Work out the finished part from the listing and answer in its coordinate system (mm). A direction names the side the tool comes from. Give positions to 0.01 mm unless a question says otherwise; leave off trailing zeros. Write each loop counter-clockwise with the first axis right and the second up, starting at its lowest first coordinate (ties: lowest second). Pieces come first, ordered by that corner, then holes. Notation, with made-up numbers: (-20, 46) -> (2, 46) arc R21 cw to (2, 75) -> close; hole circle Ø4 at (56, 3). An arc over 180 degrees is marked (long way). Use a Markdown table: item, result. Add a question column.
Q1. Section A-A, the plane y = 94.5 is taken. Give the vertices of the cut face in (x, z).
Q2. For faces 5 (the face through (0, 50, 0)), 6 (the face through (0, 55, 0)), 7 (the face through (-5.536, 10.14, 0.325)), 8 (the face through (0, 175, 8)), determine the directions among +Z, -Z, +X, -X, +Y, -Y from which every point of the face is accessible in a straight line to the end or side of a thin tool.
Q3. Consider line 1 (Z direction, x = 0, y = 69.75); line 2 (Z direction, x = 0, y = 4.5); line 3 (X direction, y = 84.5, z = 0.5). Determine where each line is inside the solid, lowest interval first.
Q4. For a pull along X with two mould halves and no side action, classify faces 1 (the face through (-2, 55, 6)), 2 (the face through (-1.08, 34.79, -4.88)), 3 (the face through (0, 0, 0)), 4 (the face through (1, 75, -5)) as pulls with the +X half, pulls with the -X half, needs draft (parallel to the pull), parting line crosses it, or undercut.
Q5. Each of these flat-tipped pins is pushed along its axis until it touches: pin 1 Ø1.8 at (x, z) = (0.5, 0.5) entering from +Y; pin 2 Ø10 at (y, z) = (132.5, -8.5) entering from -X; pin 3 Ø1.5 at (x, y) = (-1.5, 44) entering from -Z. Where does it stop, or does it pass through?
Autodesk Inventor part; units mm, degrees
ref_plane "YZ Plane" through (0, 0, 0) normal (1, 0, 0) x (0, 1, 0)
ref_plane "XZ Plane" through (0, 0, 0) normal (0, 1, 0) x (-1, 0, 0)
ref_plane "XY Plane" through (0, 0, 0) normal (0, 0, 1) x (1, 0, 0)
sketch "Sketch1" plane through (0, 0, 0) normal (0, 1, 0) x (-1, 0, 0)
  ellipse E0 centre (0, 0) end of major axis (0, 11.8) minor radius 4.3
  ellipse E1 centre (0, 0) end of major axis (11.8, 0) minor radius 4.3
  dimension "d0" = 11.8
  dimension "d1" = 4.3
  dimension "d2" = 11.8
  dimension "d3" = 4.3
sketch "Sketch2" plane through (0, 0, 0) normal (0, 1, 0) x (-1, 0, 0)
  circle A0 centre (7, 0) radius 1.5
  circle A1 centre (0, -7) radius 1.5
  circle A2 centre (-7, 0) radius 1.5
  circle A3 centre (0, 7) radius 1.5
  point P0 (0, 0)
  dimension "d4" = 3
  dimension "d5" = 3
  dimension "d6" = 3
  dimension "d7" = 3
  dimension "d8" = 7
  dimension "d9" = 7
  dimension "d10" = 7
  dimension "d11" = 7
extrude "Extrusion1" add sketch "Sketch1" along normal blind 20
hole "Hole1" at (7, 0, 0) at (0, 0, 7) at (0, 0, -7) at (-7, 0, 0) direction (0, 1, 0) diameter 3 depth 20 tip angle 118
sketch "Sketch5" plane through (0, 20, 0) normal (0, 1, 0) x (1, 0, 0)
  circle A0 centre (0, 0) radius 5
  circle A1 centre (0, 0) radius 3
  dimension "d25" = 10
  dimension "d26" = 6
extrude "Extrusion3" add sketch "Sketch5" along normal blind 30
sketch "Sketch6" plane through (0, 50, 0) normal (0, 1, 0) x (1, 0, 0)
  point P0 (0, 0)
sketch "Sketch7" plane through (0, 50, 0) normal (0, 1, 0) x (1, 0, 0)
  circle A0 centre (0, 0) radius 8
  dimension "d29" = 16
extrude "Extrusion4" add sketch "Sketch7" along normal blind 5
fillet "Fillet1" radius 6.7625 1 edges at (-8, 50, 0)
sketch "Sketch8" plane through (0, 55, 0) normal (0, 1, 0) x (1, 0, 0)
  circle A0 centre (0, 0) radius 8.5
  circle A1 centre (0, 0) radius 7.5
  dimension "d33" = 17
  dimension "d34" = 15
sketch "Sketch9" plane through (0, 55, 0) normal (0, 1, 0) x (1, 0, 0)
  circle A0 centre (0, 0) radius 5.75
  circle A1 centre (0, 0) radius 4.75
  dimension "d35" = 11.5
  dimension "d36" = 9.5
extrude "Extrusion5" add sketch "Sketch8" along normal blind 120
extrude "Extrusion6" add sketch "Sketch9" along normal blind 20
sketch "Sketch10" plane through (0, 75, 0) normal (0, 1, 0) x (1, 0, 0)
  point P0 (0, 0)
sketch "Sketch11" plane through (0, 75, 0) normal (0, 1, 0) x (1, 0, 0)
  point P0 (0, 0)
fillet "Fillet4" radius 2 1 edges at (-8.5, 55, 0)
properties part number "BB-8_headslider_stilt"
Result set:
| question | item | result |
|---|---|---|
| 1 | outline | circle Ø17 at (0, 0); hole circle Ø15 at (0, 0) |
| 2 | face 5 | none |
| 2 | face 6 | +Y |
| 2 | face 7 | -Y |
| 2 | face 8 | +Z, -Z, +X, -X, +Y |
| 3 | line 1 | z = -8.5 to -7.5, -5.75 to -4.75, 4.75 to 5.75, 7.5 to 8.5 |
| 3 | line 2 | z = -11.8 to -8.5, -5.5 to 5.5, 8.5 to 11.8 |
| 3 | line 3 | x = -8.49 to -7.48, 7.48 to 8.49 |
| 4 | face 1 | undercut |
| 4 | face 2 | parting line crosses it |
| 4 | face 3 | needs draft |
| 4 | face 4 | undercut |
| 5 | pin 1 | stops at y = 55 |
| 5 | pin 2 | stops at x = -7.75 |
| 5 | pin 3 | stops at z = -4.94 |
